Geometry: see drawing. Coordinates: mm, zero at the bounding-box minimum. Coordinates: 2 decimals unless noted, no trailing zeros. Write each loop counter-clockwise with the first axis right and the second up, starting at its lowest first coordinate (ties: lowest second). Pieces come first, ordered by that corner, then holes. Notation, with made-up numbers: M -19,8.25 L -8,8.25 A32 ccw -8,35.25 Z; hole C 1.25,48 d3. An arc over 180 degrees is marked long. Write item = value, one per line. Start each with the question number.
1. Section query B-B (y = 4). Output: boundary loops of the cut face in (x, z) (1 decimal), then the cut area to 3 significant figures.
2. Section query A-A (x = 76.2). Output: boundary loops of the cut face in (y, z) (1 decimal).
3. Section query D-D (y = 26). Output: boundary loops of the cut face in (x, z) (3 decimals), then the cut area to 3 significant figures.
4. Section query C-C (z = 1.6). Give the number of separate pieces and of enclosed holes in the cut face, then the cut area to 3 significant figures.
5. Line query: line 1 along Y through (x, z) = (76.2, 2.55) (1 decimal); line 2 along Y through (x, z) = (60, 0.7) (3 decimals); line 3 along Y through (x, z) = (41, 2.85). Output: solid intervals per line, ascending.
6. Pin query (flat end, axial travel): pin 1 Ø1 at (x, z) = (70, 1) entering from +Y (3 decimals); pin 2 Ø2.5 at (x, y) = (22.225, 11.875) entering from +Z. Return the tip coordinate at first contact, or that it passes through.
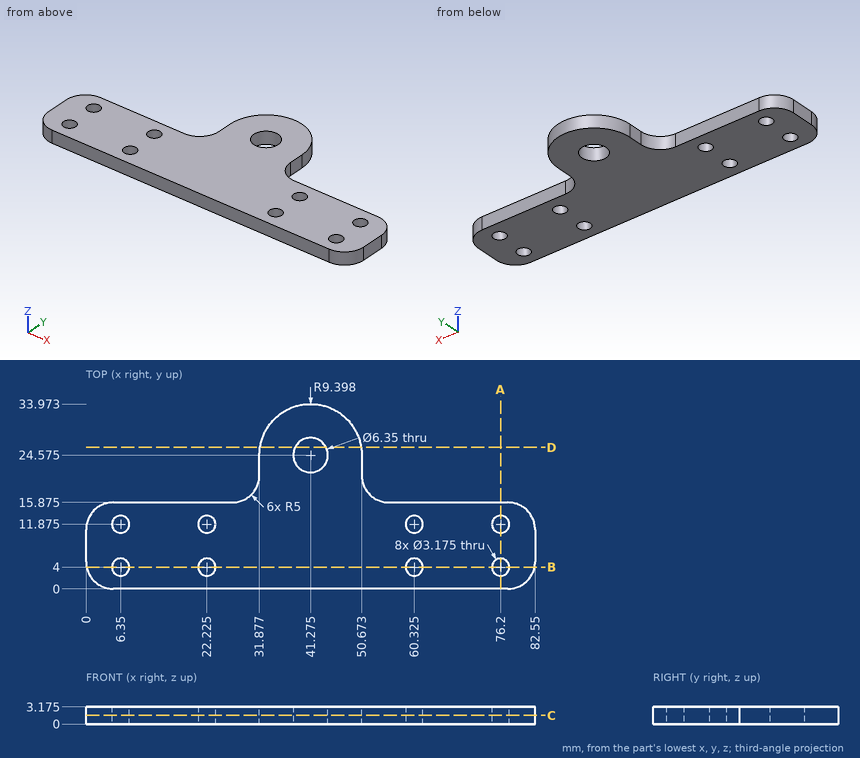
Results are:
q1.outline = M 0.1,0 L 4.8,0 L 4.8,3.2 L 0.1,3.2 Z; M 7.9,0 L 20.6,0 L 20.6,3.2 L 7.9,3.2 Z; M 23.8,0 L 58.7,0 L 58.7,3.2 L 23.8,3.2 Z; M 61.9,0 L 74.6,0 L 74.6,3.2 L 61.9,3.2 Z; M 77.8,0 L 82.4,0 L 82.4,3.2 L 77.8,3.2 Z
q1.area = 221 mm^2
q2.outline = M 0,0 L 2.4,0 L 2.4,3.2 L 0,3.2 Z; M 5.6,0 L 10.3,0 L 10.3,3.2 L 5.6,3.2 Z; M 13.5,0 L 15.9,0 L 15.9,3.2 L 13.5,3.2 Z
q3.outline = M 31.986,0 L 38.438,0 L 38.438,3.175 L 31.986,3.175 Z; M 44.112,0 L 50.564,0 L 50.564,3.175 L 44.112,3.175 Z
q3.area = 41.0 mm^2
q4.separate_pieces = 1
q4.enclosed_holes = 9
q4.area = 1,510 mm^2
q5.line_1 = 0 to 2.4, 5.6 to 10.3, 13.5 to 15.9
q5.line_2 = 0 to 2.446, 5.554 to 10.321, 13.429 to 15.875
q5.line_3 = 0 to 21.41, 27.74 to 33.97
q6.pin_1 = 15.875
q6.pin_2 = through
